Here's how the part is built. I have some questions about the finished solid (model axes, mm). A direction names the side the tool comes from. Round coordinates to 2 decimals unless told otherwise and drop trailing zeros. Order: outer loops, then holes, each group sorted by start corner. A loop starts at its lowest first (then second) coordinate and runs counter-clockwise, first axis right, second up. Notation, with made-up numbers: (64.5, 56) -> (103.5, 56) arc R25 cw to (103.5, 80) -> close; hole circle Ø3 at (17.25, 83.25). An arc over 180 degrees is marked (long way). Use a Markdown table: item, result. Add a question column.
(1) I want a section at A-A, the plane x = 0. Please give me the cut outline in (y, z).
(2) Thinking about a two-plate mould opening in Z: for faces 1 (the face through (0, -7, 3)), 2 (the face through (1.908, -9.153, -0.617)), 3 (the face through (4.736, 4.313, 0.296)), which applies, pulls with the +Z half, pulls with the -Z half, needs draft (parallel to the pull), parting line crosses it, or undercut?
(3) On a 3-axis mill with a long thin cutter (end or side, diameter ignored), from which of +Z, -Z, +X, -X, +Y, -Y can I reach the whole of each face in a straight line? I mean faces 4 (the face through (0.1, 5.5, 3.3)), 5 (the face through (-4.716, 4.414, 0.296)), 6 (the face through (-0.735, -5.451, 3.154)). Say none if no direction works.
(4) I want a section at B-B, the plane y = -2.5. Please give me the cut outline in (x, z), then the cut area to 3 significant figures.
(5) If I drill on probe 1 along X at (y, z) = (1.5, 2); probe 2 along X at (y, z) = (-3, 0.5); probe 3 along Y at (x, z) = (0.25, -1.5), over which ranges is the centre line in solid material (lowest first)?
(6) I want a section at C-C, the plane z = -0.5. Please give me the cut outline in (x, y).
(7) I want a section at D-D, the plane x = 3. Please give me the cut outline in (y, z).
(8) I'm going to push a flat-ended pin straight in: P1, Ø4.5, axis at x = -3.5, y = -10, coming from the +Z side. Where does the tip first touch, or does it pass through?
from build123d import *

# Parameters (mm, degrees)
BOSS_EXTRUDE1_DEPTH          = 3
SKETCH1_R                    = 2
BOSS_EXTRUDE1_2_DEPTH        = 3
BOSS_EXTRUDE4_START          = 3.5
BOSS_EXTRUDE4_DEPTH          = 6.5
F_4_0_4_DIAMETER_HOLE1_D     = 4
F_4_0_4_DIAMETER_HOLE1_DEPTH = 15


with BuildPart() as part:
    # Sketch1 → Boss-Extrude1 (new, symmetric)
    with BuildSketch(Plane.XY):
        with BuildLine():
            Line((-5.5, 0), (-14.456832294800959, -4))
            ThreePointArc((-14.45683229480096, -4.000000000000001), (1.78e-15, -15), (14.456832294800964, -4))
            Line((14.456832294800959, -4), (5.5, 0))
            ThreePointArc((5.5, -1.35e-15), (3.8890872965259793, -3.8890872965260432), (-8.406e-14, -5.5))
            ThreePointArc((-8.406e-14, -5.5), (-3.8890872965260415, -3.8890872965259815), (-5.5, 6.7e-16))
        make_face()
    extrude(amount=BOSS_EXTRUDE1_DEPTH, both=True)



with BuildPart() as body_2:
    # Sketch1 → Boss-Extrude1 2 (new, symmetric)
    with BuildSketch(Plane.XY):
        with BuildLine():
            Line((-4, 8), (-5.313044131475103, 1.4218164638932054))
            ThreePointArc((-5.313044131475121, 1.4218164638932076), (-6.7e-16, 5.5), (5.313044131475121, 1.421816463893209))
            Line((5.313044131475103, 1.4218164638932063), (4, 8))
            ThreePointArc((4, 8), (2e-17, 12), (-4, 8))
        make_face()
        with Locations((8.9e-16, 8)):
            Circle(SKETCH1_R, mode=Mode.SUBTRACT)
    extrude(amount=BOSS_EXTRUDE1_2_DEPTH, both=True)


with BuildPart() as part_1:
    add(part.part)

    add(body_2.part)  # Boss-Extrude4 merges body 2
    # Sketch1<5> → Boss-Extrude4 (add)
    with BuildSketch(Plane.XY.offset(BOSS_EXTRUDE4_START)):
        with BuildLine():
            Line((0, -4), (0, -5.5))
            ThreePointArc((-8.406e-14, -5.5), (3.8890872965259793, -3.8890872965260432), (5.5, -1.35e-15))
            ThreePointArc((5.5, 0), (5.487925108620274, 0.3642499171930612), (5.45175345375449, 0.7269004605006023))
            Line((5.45175345375449, 0.7269004605006018), (5.313044131475103, 1.4218164638932063))
            ThreePointArc((5.31304413147512, 1.421816463893209), (3.348881115282156, 4.362911330259479), (-8.271e-14, 5.5))
            Line((0, 5.500000000000002), (0, 4))
            ThreePointArc((-1.2321e-13, 4), (2.8284271247461463, 2.828427124746234), (4, 0))
            ThreePointArc((4, -9.8e-16), (2.8284271247461468, -2.8284271247462334), (-1.2508e-13, -4))
        make_face()
        with BuildLine():
            ThreePointArc((-5.45175345375449, 0.7269004605006025), (-5.487925108620274, 0.36424991719306166), (-5.5, 6.7e-16))
            ThreePointArc((-5.5, 6.7e-16), (-3.8890872965260415, -3.8890872965259815), (-8.406e-14, -5.5))
            Line((0, -5.5), (0, -4))
            ThreePointArc((-1.2508e-13, -4), (-4, 4.9e-16), (-1.2321e-13, 4))
            Line((0, 4), (0, 5.500000000000002))
            ThreePointArc((-8.271e-14, 5.5), (-3.3488811152822207, 4.36291133025943), (-5.31304413147512, 1.4218164638932085))
            Line((-5.313044131475103, 1.4218164638932054), (-5.45175345375449, 0.7269004605006018))
        make_face()
    extrude(amount=-BOSS_EXTRUDE4_DEPTH)

    # Ø4.0 (4) Diameter Hole1
    with Locations(Plane(origin=(0, -15, -0.016063309), x_dir=(-1, 0, 0), z_dir=(0, -1, 0))):
        with Locations((0, 0)):
            Hole(F_4_0_4_DIAMETER_HOLE1_D / 2, depth=F_4_0_4_DIAMETER_HOLE1_DEPTH)


solid = part_1.part
Taken from the geometry:
| question | item | result |
|---|---|---|
| 1 | outline | (-15, -3) -> (-4, -3) -> (-4, -2.02) -> (-15, -2.02) -> close; (-15, 1.98) -> (-4, 1.98) -> (-4, 3.5) -> (-5.5, 3.5) -> (-5.5, 3) -> (-15, 3) -> close; (4, -3) -> (6, -3) -> (6, 3) -> (5.5, 3) -> (5.5, 3.5) -> (4, 3.5) -> close; (10, -3) -> (12, -3) -> (12, 3) -> (10, 3) -> close |
| 2 | face 1 | pulls with the +Z half |
| 2 | face 2 | undercut |
| 2 | face 3 | needs draft |
| 3 | face 4 | +Z, +Y |
| 3 | face 5 | +Z, -Z, -X, +Y |
| 3 | face 6 | +Z |
| 4 | outline | (-11.1, -3) -> (-3.12, -3) -> (-3.12, 3.5) -> (-4.9, 3.5) -> (-4.9, 3) -> (-11.1, 3) -> close; (3.12, -3) -> (11.1, -3) -> (11.1, 3) -> (4.9, 3) -> (4.9, 3.5) -> (3.12, 3.5) -> close |
| 4 | area | 97.5 mm2 |
| 5 | probe 1 | x = -5.3 to -3.71, 3.71 to 5.3 |
| 5 | probe 2 | x = -12.22 to -2.65, 2.65 to 12.22 |
| 5 | probe 3 | y = 3.99 to 6.02, 9.98 to 11.99 |
| 6 | outline | (-14.46, -4) arc R15 ccw to (-1.94, -14.87) -> (-1.94, -3.5) arc R4 cw (long way) to (1.94, -3.5) -> (1.94, -14.87) arc R15 ccw to (14.46, -4) -> (5.5, 0) arc R5.5 ccw to (5.45, 0.73) -> (4, 8) arc R4 ccw to (-4, 8) -> (-5.45, 0.73) arc R5.5 ccw to (-5.5, 0) -> close; hole circle Ø4 at (0, 8) |
| 7 | outline | (-14.7, -3) -> (-2.65, -3) -> (-2.65, 3.5) -> (-4.61, 3.5) -> (-4.61, 3) -> (-14.7, 3) -> close; (2.65, -3) -> (10.65, -3) -> (10.65, 3) -> (4.61, 3) -> (4.61, 3.5) -> (2.65, 3.5) -> close |
| 8 | P1 | stops at z = 3 |
